Can you work these out from the model? Positions are in its coordinate system, mm. A direction names the side the tool comes from. Coordinates: 2 decimals unless noted, no trailing zeros. Write each loop counter-clockwise with the first axis right and the second up, starting at its lowest first coordinate (ties: lowest second). Pieces come first, ordered by that corner, then holes. Notation, with made-up numbers: (24, -31) - (62, -31) arc R13 cw to (62, -23) - close; hole circle Ø7 at (34.25, -4). An arc over 180 degrees is marked (long way). Use one line per item in the form item = value. Start each with the question number.
(1) On a 3-axis mill with a long thin cutter (end or side, diameter ignored), from which of +Z, -Z, +X, -X, +Y, -Y can I reach the whole of each face in a straight line? I mean faces 1 (the face through (6.14, -1.78, 0.6)), 2 (the face through (11.6, -5, 7.4)), 3 (the face through (5, 18, 7)), 4 (the face through (8.56, 40.97, 14.4)). Say none if no direction works.
(2) If we section it at A-A on y = 15.5: Please give me the cut outline in (x, z), then the cut area to 3 significant figures.
(3) Thinking about a two-plate mould opening in X: for faces 5 (the face through (2, 9, 0)), 6 (the face through (6.16, -1.81, 14.4)), 7 (the face through (10.536, 43.249, 7.423)), which applies, pulls with the +X half, pulls with the -X half, needs draft (parallel to the pull), parting line crosses it, or undercut?
(4) For pin 1 Ø3.5 at (y, z) = (20, 9.5) entering from +X; pin 2 Ø8 at (x, z) = (8, 11.5) entering from +Y; pin 3 Ø6 at (x, z) = (19, 10.5) entering from +Y; pin 4 Ø12 at (x, y) = (7, 13) entering from -Z, each with a flat end and sliding along its axis, tell me the tip position at first contact or that it passes through.
(5) If I drill on probe 1 along Y at (x, z) = (1, 7.5); probe 2 along Y at (x, z) = (1.2, 7.5); probe 3 along Z at (x, y) = (4.5, 34), over which ranges is the centre line in solid material (lowest first)? Write a range as from..to.
Autodesk Fusion 360 part; units mm, degrees
sketch "Sketch1" plane through (0, 0, 0) normal (0, 0, 1) x (1, 0, 0)
  line L0 (11.547, 55) -> (0, 35)
  line L1 (0, 35) -> (0, 0)
  line L2 (0, 0) -> (5.4848, -9.5)
  line L3 (17.6092, -9.5) -> (23.094, 0)
  line L4 (15.8771, 52.5) -> (5, 33.6603)
  line L5 (5, 33.6603) -> (5, 1.3397)
  line L6 (5, 1.3397) -> (7.2169, -2.5)
  line L7 (15.8771, -2.5) -> (18.7639, 2.5)
  line L8 (15.8771, 52.5) -> (11.547, 55)
  line L9 (23.094, 0) -> (18.7639, 2.5)
  arc A0 (7.2169, -2.5) -> (15.8771, -2.5) centre (11.547, 0) ccw
  arc A1 (5.4848, -9.5) -> (17.6092, -9.5) centre (11.547, -6) ccw
  point P0 (11.547, -20)
  dimension "d1" = 35
  dimension "d2" = 20
  dimension "d3" = 20
  dimension "d4" = 20
  dimension "d5" = 150
  dimension "d6" = 150
  dimension "d8" = 5
  dimension "d9" = 7
sketch "Sketch2" plane through (0, 0, 0) normal (0, 0, 1) x (1, 0, 0)
sketch "Sketch3" plane through (0, 0, 0) normal (0, 0, 1) x (1, 0, 0)
sketch "Sketch4" plane through (0, 0, 0) normal (0, 0, 1) x (1, 0, 0)
sketch "Sketch5" plane through (0, 0, 0) normal (0, 0, 1) x (1, 0, 0)
sketch "Sketch6" plane through (0, 0, 0) normal (0, 0, 1) x (1, 0, 0)
sketch "Sketch7" plane through (0, 0, 0) normal (0, 0, 1) x (1, 0, 0)
sketch "Sketch8" plane through (0, 0, 0) normal (0, 0, 1) x (1, 0, 0)
extrude "Extrude1" add sketch "Sketch1" along normal blind 15
sketch "Sketch9" plane through (5, 0, 0) normal (1, 0, 0) x (0, 0, -1)
  line L0 (0, 1.3397) -> (0, 33.6603)
  line L1 (0, 33.6603) -> (-15, 33.6603)
  line L2 (-15, 33.6603) -> (-15, 1.3397)
  line L3 (-15, 1.3397) -> (0, 1.3397)
  line L4 (-7.5, 33.6603) -> (-7.5, 1.3397) construction
  line L5 (0, 17.5) -> (-15, 17.5) construction
  circle A0 centre (-7.5, 25.6603) radius 4
  circle A1 centre (-7.5, 9.3397) radius 4
  dimension "d12" = 8
  dimension "d13" = 8
extrude "Extrude2" cut sketch "Sketch9" against normal blind 3 draft -35 contours A0 | A1
extrude "Extrude3" cut 2 faces at (2, 25.2296, 7.9641) (2, 8.5998, 6.9769) along direction (-1, 0, 0) through all
fillet "Fillet1" radius 7.5 4 edges at (13.7121, 53.75, 15) (13.7121, 53.75, 0) (20.9289, 1.25, 15) (20.9289, 1.25, 0)
fillet "Fillet2" radius 8 4 edges at (5, 33.6603, 7.5) (5, 1.3397, 7.5) (0, 0, 7.5) (0, 35, 7.5)
fillet "Fillet3" radius 2 16 edges at (5.2726, 33.5872, 15) (9.0995, 40.7607, 15) (15.8771, 52.5, 7.5) (9.0995, 40.7607, 0) (5.2726, 33.5872, 0) (5, 17.5, 0) (5.2726, 1.4128, 0) (6.6443, -1.5083, 0) (10.6702, -4.9225, 0) (15.3815, -3.2072, 0.0512) (18.7639, 2.5, 7.5) (15.3815, -3.2072, 14.9488) (10.6702, -4.9225, 15) (6.6443, -1.5083, 15) (5.2726, 1.4128, 15) (5, 17.5, 15)
equation "d3 = d2"
equation "d4 = d2"
equation "d6 = d5"
Reported:
q1.face_1 = -Z
q1.face_2 = +Z, -Z
q1.face_3 = +Z, -Z, +X
q1.face_4 = +Z, +X
q2.outline = (0, 0) - (3, 0) arc R2 ccw to (5, 2) - (5, 13) arc R2 ccw to (3, 15) - (0, 15) - close
q2.area = 73.3 mm2
q3.face_5 = needs draft
q3.face_6 = undercut
q3.face_7 = pulls with the +X half
q4.pin_1 = 5
q4.pin_2 = 54.78
q4.pin_3 = 1.77
q4.pin_4 = 0
q5.probe_1 = -1.73..7.44, 11.24..23.76, 27.56..36.73
q5.probe_2 = -2.08..7.44, 11.24..23.76, 27.56..37.08
q5.probe_3 = 0.36..14.64
